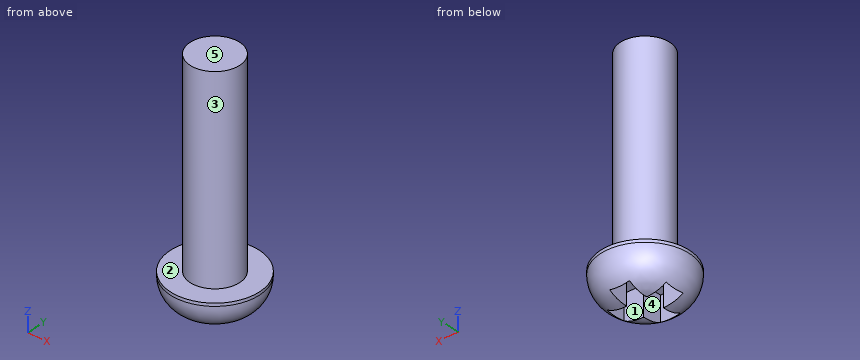
```python
from build123d import *

# Parameters (mm, degrees)
SKETCH_1_R          = 4.5
EXTRUDE_1_DEPTH     = 3.3
SKETCH_2_R          = 2.5
EXTRUDE_2_DEPTH     = 20
FILLET_2_R          = 3
SKETCH_3_W          = 2
SKETCH_3_H          = 2
CUT_EXTRUDE_1_DEPTH = 3


with BuildPart() as part:
    # ｽｹｯﾁ1 → ﾎﾞｽ - 押し出し1 (new body)
    with BuildSketch(Plane.XY):
        Circle(SKETCH_1_R)
    extrude(amount=EXTRUDE_1_DEPTH)

    # ｽｹｯﾁ2 → ﾎﾞｽ - 押し出し2 (add)
    with BuildSketch(Plane.XY.offset(3.3)):
        Circle(SKETCH_2_R)
    extrude(amount=EXTRUDE_2_DEPTH)

    # ﾌｨﾚｯﾄ2
    fillet_2_edges = [part.edges().sort_by_distance(p)[0] for p in [
        (-4.5, 0, 0),
    ]]
    fillet(fillet_2_edges, radius=FILLET_2_R)

    # ｽｹｯﾁ3 → ｶｯﾄ - 押し出し1 (cut)
    with BuildSketch(Plane(origin=(0, 0, 0), x_dir=(-1, 0, 0), z_dir=(0, 0, -1))):
        with BuildLine():
            Line((-1, 3), (-1, 1.118033989))
            ThreePointArc((-1, 1.118033989), (0, 1.5), (1, 1.118033989))
            Line((1, 1.118033989), (1, 3))
            Line((1, 3), (-1, 3))
        make_face()
        Rectangle(SKETCH_3_W, SKETCH_3_H)
        with BuildLine():
            ThreePointArc((1.5, 0), (1.401258538, -0.535233135), (1.118033989, -1))
            Line((1.118033989, -1), (3, -1))
            Line((3, -1), (3, 1))
            Line((3, 1), (1.118033989, 1))
            ThreePointArc((1.118033989, 1), (1.401258538, 0.535233135), (1.5, 0))
        make_face()
        with BuildLine():
            Line((1, 1), (1, -1))
            Line((1, -1), (1.118033989, -1))
            ThreePointArc((1.118033989, -1), (1.401258538, -0.535233135), (1.5, 0))
            ThreePointArc((1.5, 0), (1.401258538, 0.535233135), (1.118033989, 1))
            Line((1.118033989, 1), (1, 1))
        make_face()
        with BuildLine():
            ThreePointArc((-1.118033989, 1), (-1.5, 0), (-1.118033989, -1))
            Line((-1.118033989, -1), (-1, -1))
            Line((-1, -1), (-1, 1))
            Line((-1, 1), (-1.118033989, 1))
        make_face()
        with BuildLine():
            Line((-3, 1), (-3, -1))
            Line((-3, -1), (-1.118033989, -1))
            ThreePointArc((-1.118033989, -1), (-1.5, 0), (-1.118033989, 1))
            Line((-1.118033989, 1), (-3, 1))
        make_face()
        with BuildLine():
            Line((1, -1), (-1, -1))
            Line((-1, -1), (-1, -1.118033989))
            ThreePointArc((-1, -1.118033989), (0, -1.5), (1, -1.118033989))
            Line((1, -1.118033989), (1, -1))
        make_face()
        with BuildLine():
            ThreePointArc((1, -1.118033989), (0, -1.5), (-1, -1.118033989))
            Line((-1, -1.118033989), (-1, -3))
            Line((-1, -3), (1, -3))
            Line((1, -3), (1, -1.118033989))
        make_face()
        with BuildLine():
            Line((-1, 1.118033989), (-1, 1))
            Line((-1, 1), (1, 1))
            Line((1, 1), (1, 1.118033989))
            ThreePointArc((1, 1.118033989), (0, 1.5), (-1, 1.118033989))
        make_face()
    extrude(amount=-CUT_EXTRUDE_1_DEPTH, mode=Mode.SUBTRACT)


solid = part.part
```
Check sheet for the modelled part. Datum: model origin and axes. Units: mm. Face numbers are marked on the shaded views. A direction names the side the tool comes from. Coordinates: 2 decimals unless noted, no trailing zeros. Loops run counter-clockwise (first coordinate to the right, second up) from the corner with the lowest first, then second, coordinate; pieces in that order, holes last.
1) Release check for a two-part mould opening along Y. For the marked faces 1, 2 and 3 record: released by +Y, released by -Y, zero draft, split by the parting line, or undercut.
2) Gauge pin test, flat ends, axial feed: pin 1 (1.6 mm diameter, centred on x = 1.5, z = 1.5, fed in from -Y); pin 2 (2 mm diameter, centred on x = 1.5, z = 1, fed in from +Y); pin 3 (1 mm diameter, centred on x = -2.5, z = 1.5, fed in from -Y); pin 4 (2 mm diameter, centred on y = 0, z = 2.5, fed in from -X). Record the tip position at first contact, or that the pin passes through.
3) Sectioned sample at A-A (z = 14). Record the boundary of the cut face in (x, y).
4) Access from +Z, -Z, +X, -X, +Y, -Y to the whole of each face (thin tool, end or side, straight path). Record for the marked faces 4 and 5.
5) Material ranges on probe 1 along Z at (x, y) = (0, -0.5); probe 2 along Z at (x, y) = (2, -2); probe 3 along Y at (x, z) = (2, 4.25), recorded low to high.
Check sheet entries:
1. face 1: undercut
1. face 2: zero draft
1. face 3: split by the parting line
2. pin 1: stops at y = -4.25
2. pin 2: stops at y = 4.16
2. pin 3: stops at y = -3.7
2. pin 4: stops at x = -4.5
3. outline: circle Ø5 at (0, 0)
4. face 4: -Z
4. face 5: +Z, +X, -X, +Y, -Y
5. probe 1: z = 3 to 23.3
5. probe 2: z = 0.31 to 3.3
5. probe 3: y = -1.5 to 1.5
